```python
from build123d import *

# Parameters (mm, degrees)
SKETCH1_W           = 60
SKETCH1_H           = 100
BOSS_EXTRUDE1_DEPTH = 5
SKETCH2_R           = 2.5
CUT_EXTRUDE1_DEPTH  = 5
BOSS_EXTRUDE2_DEPTH = 5
SKETCH6_R           = 7.5
CUT_EXTRUDE3_DEPTH  = 5
SKETCH7_W           = 60
SKETCH7_H           = 5
BOSS_EXTRUDE3_DEPTH = 60
SKETCH8_R           = 1.75
SKETCH8_W           = 21
SKETCH8_H           = 41
CUT_EXTRUDE5_DEPTH  = 30
FILLET1_R           = 15
SKETCH13_R          = 2.5
CUT_EXTRUDE7_DEPTH  = 10
SKETCH15_R          = 2.5
CUT_EXTRUDE8_DEPTH  = 10
SKETCH16_W          = 25
SKETCH16_H          = 40
CUT_EXTRUDE9_DEPTH  = 10
FILLET3_R           = 10
SKETCH17_R          = 2.5
CUT_EXTRUDE10_DEPTH = 10
SKETCH18_W          = 2.5
SKETCH18_H          = 10
CUT_EXTRUDE11_DEPTH = 1.5


with BuildPart() as part:
    # Sketch1 → Boss-Extrude1 (new body)
    with BuildSketch(Plane(origin=(0, 0, 0), x_dir=(1, 0, 0), z_dir=(0, 1, 0))):
        Rectangle(SKETCH1_W, SKETCH1_H)
    extrude(amount=BOSS_EXTRUDE1_DEPTH)

    # Sketch2 → Cut-Extrude1 (cut)
    with BuildSketch(Plane(origin=(0, 5, 0), x_dir=(1, 0, 0), z_dir=(0, 1, 0))):
        with Locations(Location((0, 40, 0), (0, 0, 270))):
            Circle(SKETCH2_R)
        with Locations(Location((10, 40, 0), (0, 0, 270))):
            Circle(SKETCH2_R)
        with Locations(Location((20, 40, 0), (0, 0, 270))):
            Circle(SKETCH2_R)
        with Locations(Location((-20, 40, 0), (0, 0, 90))):
            Circle(SKETCH2_R)
        with Locations(Location((-10, 40, 0), (0, 0, 90))):
            Circle(SKETCH2_R)
    extrude(amount=-CUT_EXTRUDE1_DEPTH, mode=Mode.SUBTRACT)

    # Sketch5 → Boss-Extrude2 (add)
    with BuildSketch(Plane(origin=(0, 5, 0), x_dir=(1, 0, 0), z_dir=(0, 1, 0))):
        with BuildLine():
            Line((0, -50), (-30, -50))
            ThreePointArc((-30, -50), (-29.173280954, -60.651847283), (-29.77329768, -71.318866307))
            ThreePointArc((-29.77329768, -71.318866307), (0, -105), (29.77329768, -71.318866307))
            ThreePointArc((29.77329768, -71.318866307), (29.173280954, -60.651847283), (30, -50))
            Line((30, -50), (0, -50))
        make_face()
    extrude(amount=-BOSS_EXTRUDE2_DEPTH)

    # Sketch6 → Cut-Extrude3 (cut)
    with BuildSketch(Plane(origin=(0, 5, 0), x_dir=(1, 0, 0), z_dir=(0, 1, 0))):
        with Locations(Location((0, -75, 0), (0, 0, 270))):
            Circle(SKETCH6_R)
    extrude(amount=-CUT_EXTRUDE3_DEPTH, mode=Mode.SUBTRACT)

    # Sketch7 → Boss-Extrude3 (add)
    with BuildSketch(Plane(origin=(0, 5, 0), x_dir=(1, 0, 0), z_dir=(0, 1, 0))):
        with Locations((0, -28.53)):
            Rectangle(SKETCH7_W, SKETCH7_H)
    extrude(amount=BOSS_EXTRUDE3_DEPTH)

    # Sketch8 → Cut-Extrude5 (cut)
    with BuildSketch(Plane.XY.offset(31.03)):
        with Locations((-5.85, 59.35)):
            Circle(SKETCH8_R)
        with Locations((5.85, 59.35)):
            Circle(SKETCH8_R)
        with Locations((5.85, 10.65)):
            Circle(SKETCH8_R)
        with Locations((-5.85, 10.65)):
            Circle(SKETCH8_R)
        with Locations((0, 35)):
            Rectangle(SKETCH8_W, SKETCH8_H)
    extrude(amount=-CUT_EXTRUDE5_DEPTH, mode=Mode.SUBTRACT)

    # Fillet1
    fillet1_edges = [part.edges().sort_by_distance(p)[0] for p in [
        (30, 65, 28.53),
        (-30, 65, 28.53),
    ]]
    fillet(fillet1_edges, radius=FILLET1_R)

    # Sketch13 → Cut-Extrude7 (cut)
    with BuildSketch(Plane(origin=(0, 5, 0), x_dir=(1, 0, 0), z_dir=(0, 1, 0))):
        with Locations(Location((-20, 25, 0), (0, 0, 270))):
            Circle(SKETCH13_R)
        with Locations(Location((-20, 10, 0), (0, 0, 270))):
            Circle(SKETCH13_R)
        with Locations(Location((-20, -5, 0), (0, 0, 270))):
            Circle(SKETCH13_R)
        with Locations(Location((20, -5, 0), (0, 0, 90))):
            Circle(SKETCH13_R)
        with Locations(Location((20, 10, 0), (0, 0, 90))):
            Circle(SKETCH13_R)
        with Locations(Location((20, 25, 0), (0, 0, 90))):
            Circle(SKETCH13_R)
    extrude(amount=-CUT_EXTRUDE7_DEPTH, mode=Mode.SUBTRACT)

    # Sketch15 → Cut-Extrude8 (cut)
    with BuildSketch(Plane(origin=(0, 5, 0), x_dir=(1, 0, 0), z_dir=(0, 1, 0))):
        with Locations(Location((-20, -20, 0), (0, 0, 270))):
            Circle(SKETCH15_R)
        with Locations(Location((-10, -20, 0), (0, 0, 270))):
            Circle(SKETCH15_R)
        with Locations(Location((0, -20, 0), (0, 0, 270))):
            Circle(SKETCH15_R)
        with Locations(Location((10, -20, 0), (0, 0, 270))):
            Circle(SKETCH15_R)
        with Locations(Location((20, -20, 0), (0, 0, 270))):
            Circle(SKETCH15_R)
    extrude(amount=-CUT_EXTRUDE8_DEPTH, mode=Mode.SUBTRACT)

    # Sketch16 → Cut-Extrude9 (cut)
    with BuildSketch(Plane(origin=(0, 5, 0), x_dir=(1, 0, 0), z_dir=(0, 1, 0))):
        with Locations((0, 11.985)):
            Rectangle(SKETCH16_W, SKETCH16_H)
    extrude(amount=-CUT_EXTRUDE9_DEPTH, mode=Mode.SUBTRACT)

    # Fillet3
    fillet3_edges = [part.edges().sort_by_distance(p)[0] for p in [
        (-30, 2.5, -50),
        (30, 2.5, -50),
    ]]
    fillet(fillet3_edges, radius=FILLET3_R)

    # Sketch17 → Cut-Extrude10 (cut)
    with BuildSketch(Plane(origin=(0, 5, 0), x_dir=(1, 0, 0), z_dir=(0, 1, 0))):
        with Locations(Location((0, -57.5, 0), (0, 0, 270))):
            Circle(SKETCH17_R)
        with Locations(Location((17.5, -75, 0), (0, 0, 270))):
            Circle(SKETCH17_R)
        with Locations(Location((0, -92.5, 0), (0, 0, 270))):
            Circle(SKETCH17_R)
        with Locations(Location((-17.5, -75, 0), (0, 0, 270))):
            Circle(SKETCH17_R)
    extrude(amount=-CUT_EXTRUDE10_DEPTH, mode=Mode.SUBTRACT)

    # Sketch18 → Cut-Extrude11 (cut)
    with BuildSketch(Plane(origin=(0, 0, 26.03), x_dir=(-1, 0, 0), z_dir=(0, 0, -1))):
        with Locations((0, 60)):
            Rectangle(SKETCH18_W, SKETCH18_H)
        with Locations((0, 10)):
            Rectangle(SKETCH18_W, SKETCH18_H)
    extrude(amount=-CUT_EXTRUDE11_DEPTH, mode=Mode.SUBTRACT)


solid = part.part
```
Input: part model. Units: mm. Frame: model coordinates. A direction names the side the tool comes from. Coordinates: 2 decimals unless noted, no trailing zeros. Write each loop counter-clockwise with the first axis right and the second up, starting at its lowest first coordinate (ties: lowest second). Pieces come first, ordered by that corner, then holes. Notation, with made-up numbers: (24.5, 56.25) -> (31.5, 56.25) arc R11 ccw to (31.5, 64.25) -> close; hole circle Ø7 at (62.25, 75.25). An arc over 180 degrees is marked (long way). Answer as a JSON object with one key per item and string values.
1. Mould query, pull axis Z, two halves, no side actions, for faces 1 (the face through (-14, 35, 31.03)), 2 (the face through (10.5, 35, 29)), 3 (the face through (29.17, 2.54, 60.8)). Classes: released by +Z, released by -Z, zero draft, split by the parting line, or undercut.
Result set:
{"face 1": "released by +Z", "face 2": "zero draft", "face 3": "undercut"}
2. Section C-C on y = 10.65. Return the cut outline in (x, z), then the cut area to 3 significant figures.
Result set:
{"outline": "(-30, 26.03) -> (-7.6, 26.03) -> (-7.6, 31.03) -> (-30, 31.03) -> close; (-4.1, 26.03) -> (-1.25, 26.03) -> (-1.25, 27.53) -> (1.25, 27.53) -> (1.25, 26.03) -> (4.1, 26.03) -> (4.1, 31.03) -> (-4.1, 31.03) -> close; (7.6, 26.03) -> (30, 26.03) -> (30, 31.03) -> (7.6, 31.03) -> close", "area": "261 mm2"}
3. Access query for faces 4 (the face through (0, 55.5, 29)), 5 (the face through (0, 5, 67)), 6 (the face through (0, 3, -31.985)). Directions: +Z, -Z, +X, -X, +Y, -Y. A direction counts if a zero-diameter tool reaches every point of the face in a straight line with its end or side. Return the directions, or none.
Result set:
{"face 4": "+Z, -Z", "face 5": "+Z, +X, -X, +Y", "face 6": "+Y, -Y"}
4. Section B-B on z = -20. Return the cut outline in (x, y), then the cut area to 3 significant figures.
Result set:
{"outline": "(-30, 0) -> (-12.5, 0) -> (-12.5, 5) -> (-30, 5) -> close; (12.5, 0) -> (30, 0) -> (30, 5) -> (12.5, 5) -> close", "area": "175 mm2"}
5. Section D-D on x = -5.85. Return the cut outline in (y, z) (3 decimals), then the cut area to 3 significant figures.
Result set:
{"outline": "(0, -50) -> (5, -50) -> (5, -31.985) -> (0, -31.985) -> close; (0, 8.015) -> (5, 8.015) -> (5, 26.03) -> (8.9, 26.03) -> (8.9, 31.03) -> (5, 31.03) -> (5, 70.307) -> (0, 70.307) -> close; (0, 79.693) -> (5, 79.693) -> (5, 104.424) -> (0, 104.424) -> close; (12.4, 26.03) -> (14.5, 26.03) -> (14.5, 31.03) -> (12.4, 31.03) -> close; (55.5, 26.03) -> (57.6, 26.03) -> (57.6, 31.03) -> (55.5, 31.03) -> close; (61.1, 26.03) -> (65, 26.03) -> (65, 31.03) -> (61.1, 31.03) -> close", "area": "585 mm2"}
6. First-contact query: P1, Ø3, axis at x = 5.85, y = 59.35, coming from the +Z side; P2, Ø1.5, axis at x = 11.5, z = 84.5, coming from the +Y side; P3, Ø3, axis at x = -15.5, y = 19, coming from the -Z side; P4, Ø0.8, axis at x = -0.5, y = 10.5, coming from the -Z side. Flat tips, straight axial feed; report the tip coordinate or a pass-through.
Result set:
{"P1": "passes through", "P2": "stops at y = 5", "P3": "stops at z = 26.03", "P4": "stops at z = 27.53"}
7. Material intervals for line 1 (Y direction, x = -5.85, z = 28.2); line 2 (X direction, y = 1.8, z = 75); line 3 (X direction, y = 2.7, z = -25), sorted ascending. Write a range as from..to.
Result set:
{"line 1": "y = 0..8.9, 12.4..14.5, 55.5..57.6, 61.1..65", "line 2": "x = -30..-20, -15..-7.5, 7.5..15, 20..30", "line 3": "x = -30..-22.5, -17.5..-12.5, 12.5..17.5, 22.5..30"}
8. Section A-A on y = 34. Return the cut outline in (x, z), then the cut area to 3 significant figures.
Result set:
{"outline": "(-30, 26.03) -> (-10.5, 26.03) -> (-10.5, 31.03) -> (-30, 31.03) -> close; (10.5, 26.03) -> (30, 26.03) -> (30, 31.03) -> (10.5, 31.03) -> close", "area": "195 mm2"}
